```python
from build123d import *

# Parameters (mm, degrees)
SKETCH1_R           = 10.4
SKETCH1_R_2         = 0.75
SKETCH1_R_3         = 1.5
BOSS_EXTRUDE1_DEPTH = 2.3
SKETCH2_R           = 4.4
SKETCH2_R_2         = 3
BOSS_EXTRUDE2_DEPTH = 3.2


with BuildPart() as part:
    # Sketch1 → Boss-Extrude1 (new body)
    with BuildSketch(Plane(origin=(0, 0, 0), x_dir=(1, 0, 0), z_dir=(0, 1, 0))):
        Circle(SKETCH1_R)
        with Locations((7, 0)):
            Circle(SKETCH1_R_2, mode=Mode.SUBTRACT)
        with Locations((7, 3)):
            Circle(SKETCH1_R_2, mode=Mode.SUBTRACT)
        with Locations((7, -3)):
            Circle(SKETCH1_R_2, mode=Mode.SUBTRACT)
        with Locations((3, -7)):
            Circle(SKETCH1_R_2, mode=Mode.SUBTRACT)
        with Locations((0, -7)):
            Circle(SKETCH1_R_2, mode=Mode.SUBTRACT)
        with Locations((-3, -7)):
            Circle(SKETCH1_R_2, mode=Mode.SUBTRACT)
        with Locations((-7, -3)):
            Circle(SKETCH1_R_2, mode=Mode.SUBTRACT)
        with Locations((-7, 0)):
            Circle(SKETCH1_R_2, mode=Mode.SUBTRACT)
        with Locations((-7, 3)):
            Circle(SKETCH1_R_2, mode=Mode.SUBTRACT)
        with Locations((-3, 7)):
            Circle(SKETCH1_R_2, mode=Mode.SUBTRACT)
        with Locations((0, 7)):
            Circle(SKETCH1_R_2, mode=Mode.SUBTRACT)
        with Locations((3, 7)):
            Circle(SKETCH1_R_2, mode=Mode.SUBTRACT)
        Circle(SKETCH1_R_3, mode=Mode.SUBTRACT)
    extrude(amount=BOSS_EXTRUDE1_DEPTH)

    # Sketch2 → Boss-Extrude2 (add)
    with BuildSketch(Plane(origin=(0, 2.3, 0), x_dir=(1, 0, 0), z_dir=(0, 1, 0))):
        Circle(SKETCH2_R)
        Circle(SKETCH2_R_2, mode=Mode.SUBTRACT)
    extrude(amount=BOSS_EXTRUDE2_DEPTH)


solid = part.part
```
Geometry check sheet. Reference: the model listing, model coordinates, mm. A direction names the side the tool comes from. Round coordinates to 2 decimals unless told otherwise and drop trailing zeros. Loops run counter-clockwise (first coordinate to the right, second up) from the corner with the lowest first, then second, coordinate; pieces in that order, holes last. Notation, with made-up numbers: (79, 14.25) - (100, 14.25) arc R29 cw to (100, 47.25) - close; hole circle Ø2 at (3, -37.75). An arc over 180 degrees is marked (long way). Use a Markdown table: item, result.
Q1. Cross-section at B-B on x = 0. Record the cut outline in (y, z).
Solutions:
| item | result |
|---|---|
| outline | (0, -10.4) - (2.3, -10.4) - (2.3, -7.75) - (0, -7.75) - close; (0, -6.25) - (2.3, -6.25) - (2.3, -4.4) - (5.5, -4.4) - (5.5, -3) - (2.3, -3) - (2.3, -1.5) - (0, -1.5) - close; (0, 1.5) - (2.3, 1.5) - (2.3, 3) - (5.5, 3) - (5.5, 4.4) - (2.3, 4.4) - (2.3, 6.25) - (0, 6.25) - close; (0, 7.75) - (2.3, 7.75) - (2.3, 10.4) - (0, 10.4) - close |
Q2. Cross-section at D-D on z = 3.5. Record the cut outline in (x, y), plus the area to 3 significant figures.
Solutions:
| item | result |
|---|---|
| outline | (-9.79, 0) - (-7.56, 0) - (-7.56, 2.3) - (-9.79, 2.3) - close; (-6.44, 0) - (6.44, 0) - (6.44, 2.3) - (2.67, 2.3) - (2.67, 5.5) - (-2.67, 5.5) - (-2.67, 2.3) - (-6.44, 2.3) - close; (7.56, 0) - (9.79, 0) - (9.79, 2.3) - (7.56, 2.3) - close |
| area | 57.0 mm2 |
Q3. Material ranges on line 1 (Z direction, x = 0, y = 0.8); line 2 (X direction, y = 1.5, z = -2.75); line 3 (Z direction, x = 7, y = 0.6), recorded low to high.
Solutions:
| item | result |
|---|---|
| line 1 | z = -10.4 to -7.75, -6.25 to -1.5, 1.5 to 6.25, 7.75 to 10.4 |
| line 2 | x = -10.03 to -7.71, -6.29 to 6.29, 7.71 to 10.03 |
| line 3 | z = -7.69 to -3.75, -2.25 to -0.75, 0.75 to 2.25, 3.75 to 7.69 |
Q4. Go/stop test with flat-tipped pins: P1, Ø1.2, axis at x = 7, z = 0, coming from the +Y side; P2, Ø1.7, axis at x = 7, z = -3, coming from the +Y side; P3, Ø2, axis at y = 3, z = 3.5, coming from the -X side; P4, Ø3, axis at x = 3, y = 2.5, coming from the +Z side. Record where each tip stops, or that it passes through.
Solutions:
| item | result |
|---|---|
| P1 | passes through |
| P2 | stops at y = 2.3 |
| P3 | stops at x = -10.02 |
| P4 | stops at z = 10.29 |
Q5. Cross-section at C-C on z = 0. Record the cut outline in (x, y), plus the area to 3 significant figures.
Solutions:
| item | result |
|---|---|
| outline | (-10.4, 0) - (-7.75, 0) - (-7.75, 2.3) - (-10.4, 2.3) - close; (-6.25, 0) - (-1.5, 0) - (-1.5, 2.3) - (-3, 2.3) - (-3, 5.5) - (-4.4, 5.5) - (-4.4, 2.3) - (-6.25, 2.3) - close; (1.5, 0) - (6.25, 0) - (6.25, 2.3) - (4.4, 2.3) - (4.4, 5.5) - (3, 5.5) - (3, 2.3) - (1.5, 2.3) - close; (7.75, 0) - (10.4, 0) - (10.4, 2.3) - (7.75, 2.3) - close |
| area | 43.0 mm2 |
Q6. Cross-section at A-A on y = 0.8. State how many separate pieces and enclosed holes the cut face has, plus the area to 3 significant figures.
Solutions:
| item | result |
|---|---|
| separate pieces | 1 |
| enclosed holes | 13 |
| area | 312 mm2 |
Q7. Access from +Z, -Z, +X, -X, +Y, -Y to the whole of each face (thin tool, end or side, straight path). Record for faces 1 (the flat face through (4.5, 2.3, 2.2)), 2 (the cylindrical face through (-3.595, 1.134, -6.544)).
Solutions:
| item | result |
|---|---|
| face 1 | +Y |
| face 2 | +Y, -Y |
Q8. Draft check along X on faces 3 (the cylindrical face through (-1.35, 1.13, -10.31)), 4 (the cylindrical face through (-1.5, 1.13, -0.07)), 5 (the flat face through (1, 5.5, 3)). Enter one of: released by +X, released by -X, zero draft, split by the parting line, or undercut.
Solutions:
| item | result |
|---|---|
| face 3 | split by the parting line |
| face 4 | undercut |
| face 5 | zero draft |
